Source: CAD feature listing. Evaluate the final solid. Frame: model axes, mm. A direction names the side the tool comes from. Round coordinates to 2 decimals unless told otherwise and drop trailing zeros. Loops run counter-clockwise (first coordinate to the right, second up) from the corner with the lowest first, then second, coordinate; pieces in that order, holes last. Notation, with made-up numbers: (40.25, 9) -> (64.25, 9) arc R31 ccw to (64.25, 43) -> close; hole circle Ø7 at (-1, 52.25). An arc over 180 degrees is marked (long way). Put each result on its own line as item: value. Start each with the question number.
1. Contact query for flat-ended pins moving along their axis: pin 1 (0.9 mm diameter, centred on x = 2, z = 24, fed in from +Y); pin 2 (1.6 mm diameter, centred on y = 15.5, z = 2, fed in from +X); pin 3 (1.9 mm diameter, centred on y = 8, z = 12.5, fed in from +X); pin 4 (0.8 mm diameter, centred on x = 0.5, z = 13.5, fed in from -Y). Output: stop coordinate, or through.
2. Cut plane A-A (y = 15.5). Return the cut outline in (x, z).
3. Cut plane B-B (x = -0.9). Return the cut outline in (y, z), then the cut area to 3 significant figures.
4. Draft query along Z for faces 4 (the cylindrical face through (-0.76, 17.4, 24.93)), 5 (the flat face through (0.5, 11.2, 12.8)), 6 (the flat face through (-1, 0, 13)), 7 (the flat face through (0, 9, 25.5)). Return one class per face: pulls with the +Z half, pulls with the -Z half, needs draft (parallel to the pull), parting line crosses it, or undercut.
5. Material intervals for L1, parallel to Z at x = -0.95, y = 15.5; L2, parallel to Z at x = -0.1, y = 3.25; L3, parallel to X at y = 2.25, z = 16, sorted ascending.
6. Cut plane D-D (z = 18.25). Return the cut outline in (x, y).
7. Cut plane C-C (y = 7.75). Return the cut outline in (x, z), then the cut area to 3 significant figures.
8. Set-up query: faces 1 (the flat face through (1, 9, 21)), 2 (the flat face through (0, 9, 27)), 3 (the flat face through (1, 5.8, 23)). Return all of +Z, -Z, +X, -X, +Y, -Y with unobstructed straight access to the full face (end or side cutting, diameter ignored); none if empty.
Autodesk Fusion 360 part; units mm, degrees
sketch "Sketch1" plane through (0, 0, 0) normal (1, 0, 0) x (0, 1, 0)
  line L0 (0, 0) -> (18, 0)
  line L1 (18, 0) -> (18, 25.5)
  line L2 (18, 25.5) -> (0, 25.5)
  line L3 (0, 25.5) -> (0, 0)
  line L4 (5.8, 25.5) -> (12.2, 25.5)
  line L5 (12.2, 25.5) -> (12.2, 21)
  line L6 (12.2, 21) -> (5.8, 21)
  line L7 (5.8, 21) -> (5.8, 25.5)
  line L8 (9, 0) -> (9, 25.5)
  line L9 (12.2, 23.25) -> (9, 23.25)
  line L10 (5.8, 23.25) -> (9, 23.25)
  line L11 (0, 12.75) -> (18, 12.75)
  line L12 (5.8, 4.5) -> (5.8, 0)
  line L13 (5.8, 0) -> (12.2, 0)
  line L14 (12.2, 0) -> (12.2, 4.5)
  line L15 (12.2, 4.5) -> (5.8, 4.5)
  line L16 (6.8, 13.95) -> (11.2, 13.95)
  line L17 (11.2, 13.95) -> (11.2, 11.55)
  line L18 (11.2, 11.55) -> (6.8, 11.55)
  line L19 (6.8, 11.55) -> (6.8, 13.95)
  line L20 (8, 13.95) -> (8, 12.75)
  line L21 (8, 11.55) -> (8, 12.75)
  line L22 (11.2, 13.3189) -> (9, 13.3189)
  line L23 (6.8, 13.3189) -> (9, 13.3189)
  dimension "d1" = 25.5
  dimension "d2" = 18
  dimension "d3" = 6.4
  dimension "d4" = 4.5
  dimension "d5" = 4.4
  dimension "d6" = 2.4
extrude "Extrude1" add sketch "Sketch1" against normal blind 1.5
extrude "Extrude2" add sketch "Sketch1" along normal blind 2.9 contours L0 L8 L12 L13 L15 | L0 L8 L13 L14 L15 | L2 L4 L7 L8 L10 | L2 L4 L5 L8 L9 | L6 L7 L8 L10 | L5 L6 L8 L9
extrude "Extrude3" add sketch "Sketch1" along normal blind 1 contours L11 L19 L20 L23 | L11 L18 L19 L21 | L8 L11 L20 L23 | L8 L11 L18 L21 | L16 L19 L20 L23 | L8 L11 L17 L18 | L8 L11 L17 L22 | L8 L16 L20 L23 | L8 L16 L17 L22
sketch "Sketch2" plane through (0, 0, 25.5) normal (0, 0, 1) x (-1, 0, 0)
  line L0 (0, -12.2) -> (0, -18)
  line L1 (0, -18) -> (1.5, -18)
  line L2 (1.5, -18) -> (1.5, 0)
  line L3 (1.5, 0) -> (0, 0)
  line L4 (0, 0) -> (0, -5.8)
  line L5 (0, -5.8) -> (-2.9, -5.8)
  line L6 (-2.9, -5.8) -> (-2.9, -12.2)
  line L7 (-2.9, -12.2) -> (0, -12.2)
  line L8 (-2.4, -6.3) -> (-0.5, -6.3)
  line L9 (-0.5, -6.3) -> (-0.5, -11.7)
  line L10 (-0.5, -11.7) -> (-2.4, -11.7)
  line L11 (-2.4, -11.7) -> (-2.4, -6.3)
  line L12 (0, -5.8) -> (0, -12.2)
  dimension "d13" = 0.5
  dimension "d14" = 0.5
  dimension "d15" = 0.5
  dimension "d16" = 0.5
extrude "Extrude4" add sketch "Sketch2" along normal blind 0.7 contours L8 L9 L10 L11
sketch "Sketch3" plane through (0, 0, 26.2) normal (0, 0, 1) x (-1, 0, 0)
  line L0 (-2.4, -11.7) -> (-0.5, -11.7)
  line L1 (-0.5, -11.7) -> (-0.5, -6.3)
  line L2 (-0.5, -6.3) -> (-2.4, -6.3)
  line L3 (-2.4, -6.3) -> (-2.4, -11.7)
  line L4 (-2.4, -11.7) -> (-2.4, -6.3)
  line L5 (-2.4, -6.3) -> (-0.5, -6.3)
  line L6 (-0.5, -6.3) -> (-0.5, -11.7)
  line L7 (-0.5, -11.7) -> (-2.4, -11.7)
  line L8 (0, -12.2) -> (0, -18)
  line L9 (0, -18) -> (1.5, -18)
  line L10 (1.5, -18) -> (1.5, 0)
  line L11 (1.5, 0) -> (0, 0)
  line L12 (0, 0) -> (0, -5.8)
  line L13 (0, -5.8) -> (-2.9, -5.8)
  line L14 (-2.9, -5.8) -> (-2.9, -12.2)
  line L15 (-2.9, -12.2) -> (0, -12.2)
  line L16 (-2.9, -5.8) -> (0, -5.8)
  line L17 (0, -5.8) -> (0, -12.2)
  line L18 (0, -12.2) -> (-2.9, -12.2)
  line L19 (-2.9, -12.2) -> (-2.9, -5.8)
extrude "Extrude5" add sketch "Sketch3" along normal blind 1.1 contours L0 L1 L2 L3 L4 L5 L6 L7 | L13 L14 L15 L16 L17 L18 L19
sketch "Sketch4" plane through (0, 0, 0) normal (1, 0, 0) x (0, 1, 0)
  line L0 (6.8, 11.55) -> (6.8, 13.95)
  line L1 (6.8, 13.95) -> (11.2, 13.95)
  line L2 (11.2, 13.95) -> (11.2, 11.55)
  line L3 (11.2, 11.55) -> (6.8, 11.55)
  line L4 (12.2, 25.5) -> (12.2, 21)
  line L5 (12.2, 21) -> (5.8, 21)
  line L6 (5.8, 21) -> (5.8, 25.5)
  line L7 (5.8, 25.5) -> (0, 25.5)
  line L8 (0, 25.5) -> (0, 0)
  line L9 (0, 0) -> (5.8, 0)
  line L10 (5.8, 0) -> (5.8, 4.5)
  line L11 (5.8, 4.5) -> (12.2, 4.5)
  line L12 (12.2, 4.5) -> (12.2, 0)
  line L13 (12.2, 0) -> (18, 0)
  line L14 (18, 0) -> (18, 25.5)
  line L15 (18, 25.5) -> (12.2, 25.5)
  circle A0 centre (2.5, 23.5) radius 1.35
  line L16 (9, 13.95) -> (9, 20)
  line L17 (6.8, 12.75) -> (1, 12.75)
  circle A1 centre (15.5, 23.5) radius 1.35
  circle A2 centre (2.5, 2) radius 1.35
  circle A3 centre (15.5, 2) radius 1.35
  dimension "d22" = 2.7
  dimension "d23" = 2
  dimension "d24" = 2.5
extrude "Extrude6" cut sketch "Sketch4" against normal blind 4 contours A0 | A1 | A2 | A3
fillet "Fillet1" radius 2 4 edges at (-0.75, 0, 25.5) (-0.75, 18, 25.5) (-0.75, 18, 0) (-0.75, 0, 0)
Solution:
1. pin 1: stops at y = 12.2
1. pin 2: passes through
1. pin 3: stops at x = 1
1. pin 4: stops at y = 6.8
2. outline: (-1.5, 0) -> (0, 0) -> (0, 0.65) -> (-1.5, 0.65) -> close; (-1.5, 3.35) -> (0, 3.35) -> (0, 22.15) -> (-1.5, 22.15) -> close; (-1.5, 24.85) -> (0, 24.85) -> (0, 25.5) -> (-1.5, 25.5) -> close
3. outline: (0, 2) arc R2 ccw to (2, 0) -> (16, 0) arc R2 ccw to (18, 2) -> (18, 23.5) arc R2 ccw to (16, 25.5) -> (2, 25.5) arc R2 ccw to (0, 23.5) -> close; hole circle Ø2.7 at (2.5, 2); hole circle Ø2.7 at (2.5, 23.5); hole circle Ø2.7 at (15.5, 2); hole circle Ø2.7 at (15.5, 23.5)
3. area: 433 mm^2
4. face 4: pulls with the +Z half
4. face 5: undercut
4. face 6: needs draft
4. face 7: undercut
5. L1: z = 0 to 0.65, 3.35 to 22.15, 24.85 to 25.5
5. L2: z = 0 to 0.88, 3.12 to 22.38, 24.62 to 25.5
5. L3: x = -1.5 to 0
6. outline: (-1.5, 0) -> (0, 0) -> (0, 18) -> (-1.5, 18) -> close
7. outline: (-1.5, 0) -> (2.9, 0) -> (2.9, 4.5) -> (0, 4.5) -> (0, 11.55) -> (1, 11.55) -> (1, 13.95) -> (0, 13.95) -> (0, 21) -> (2.9, 21) -> (2.9, 25.5) -> (2.4, 25.5) -> (2.4, 26.2) -> (2.9, 26.2) -> (2.9, 27.3) -> (0, 27.3) -> (0, 26.2) -> (0.5, 26.2) -> (0.5, 25.5) -> (-1.5, 25.5) -> close
7. area: 71.3 mm^2
8. face 1: +X, +Y, -Y
8. face 2: +Z, -X, +Y, -Y
8. face 3: +Z, -Z, +X, -Y
